Geometry check sheet. Reference: drawing and pictorial views, mm from the part's lowest x, y, z. Round coordinates to 2 decimals unless told otherwise and drop trailing zeros. Write each loop counter-clockwise with the first axis right and the second up, starting at its lowest first coordinate (ties: lowest second). Pieces come first, ordered by that corner, then holes. Notation, with made-up numbers: (-8.75, 74.25) - (17.25, 74.25) arc R20 ccw to (17.25, 111.25) - close; hole circle Ø9 at (74.5, 40.5). An arc over 180 degrees is marked (long way). Use one line per item in the form item = value. Start each with the question number.
1) Scan lines: probe 1 along Z at (x, y) = (1.55, 186.5); probe 2 along Y at (x, z) = (4.35, 24). Record each from-to range of solid material in increasing order.
2) Gauge pin test, flat ends, axial feed: P1, Ø1, axis at x = 2, y = 35.5, coming from the -Z side; P2, Ø3, axis at x = 1, z = 121, coming from the -Y side. Record the tip position at first contact, or that the pin passes through.
3) Section check C-C (z = 41.5). Record the boundary of the cut face in (x, y), then the cut area to 3 significant figures.
4) Section check B-B (y = 79). Record the boundary of the cut face in (x, z), then the cut area to 3 significant figures.
5) Section check A-A (x = 1.8). Record the boundary of the cut face in (y, z), then the cut area to 3 significant figures.
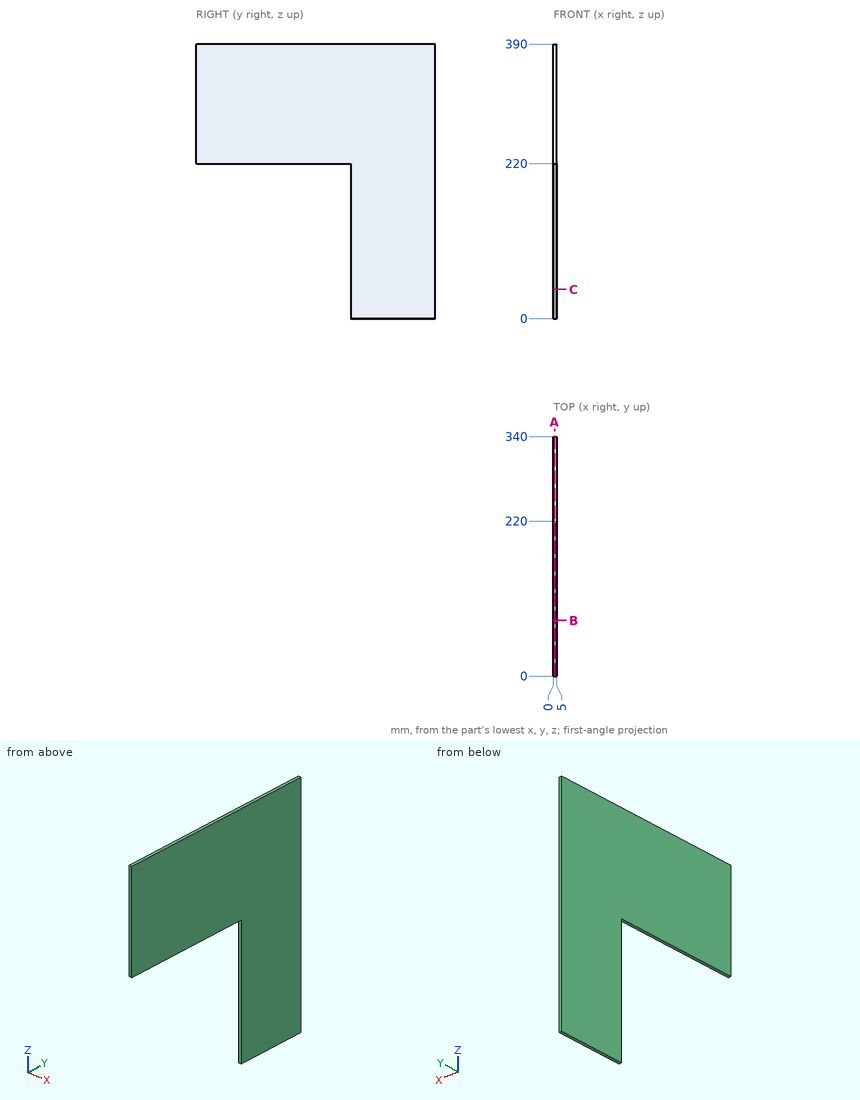
Results are:
q1.probe_1 = 220 to 390
q1.probe_2 = 220 to 340
q2.P1 = 220
q2.P2 = 220
q3.outline = (0, 220) - (5, 220) - (5, 340) - (0, 340) - close
q3.area = 600 mm²
q4.outline = (0, 220) - (5, 220) - (5, 390) - (0, 390) - close
q4.area = 850 mm²
q5.outline = (0, 220) - (220, 220) - (220, 0) - (340, 0) - (340, 390) - (0, 390) - close
q5.area = 84,200 mm²
